Read the model definition and answer for the solid it produces. Units are mm, in the model's axes. Face numbers are marked on the shaded views. A direction names the side the tool comes from. Coordinates: 2 decimals unless noted, no trailing zeros. Write each loop counter-clockwise with the first axis right and the second up, starting at its lowest first coordinate (ties: lowest second). Pieces come first, ordered by that corner, then holes.
(1) The part is cut by section B-B, the plane y = 38. State how many separate pieces and enclosed holes the cut face has, and give its area (3 significant figures).
(2) The part is cut by section A-A, the plane z = 255. Determine the outline of the cut face in (x, y), and give its area (3 significant figures).
(3) Straight lines are drawn through the part: line 1 along Z through (x, y) = (65, 22); line 2 along Z through (x, y) = (63, 25.5); line 3 along X through (y, z) = (31, 65). For each, find the intervals that lie inside material, in ascending order.
(4) Which of the six approach directions +Z, -Z, +X, -X, +Y, -Y give full straight-line access (tool end or side, diameter ignored) to the marked faces 4, 5 and 6?
(5) Given pin 1 (12 mm diameter, centred on x = 13.5, y = 34.5, fed in from -Z); pin 2 (3 mm diameter, centred on x = 95.5, y = 44, fed in from +Z); pin 3 (8 mm diameter, centred on y = 66.5, z = 295.5, fed in from +X), each flat-ended and moving along its own axis, determine where each tip first touches the part or whether it passes through.
(6) Determine the mould class of the marked faces 1, 2 and 3 for opening direction Z: pulls with the +Z half, pulls with the -Z half, needs draft (parallel to the pull), parting line crosses it, or undercut.
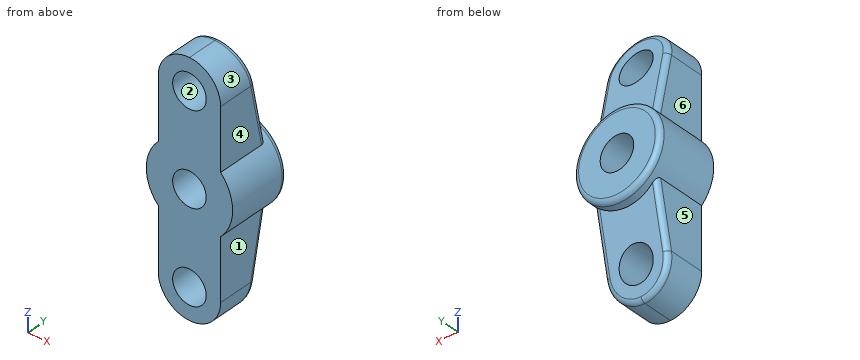
Autodesk Inventor part; units mm, degrees
ref_plane "YZ Plane" through (0, 0, 0) normal (1, 0, 0) x (0, 1, 0)
ref_plane "XZ Plane" through (0, 0, 0) normal (0, 1, 0) x (-1, 0, 0)
ref_plane "XY Plane" through (0, 0, 0) normal (0, 0, 1) x (1, 0, 0)
sketch "Sketch5" plane through (0, 0, 0) normal (1, 0, 0) x (0, 1, 0)
  line L0 (0, 0) -> (0, 510)
  line L1 (0, 510) -> (70, 510)
  line L2 (70, 510) -> (70, 0)
  line L3 (70, 0) -> (0, 0)
  line L4 (0, 255) -> (110, 255)
  line L5 (110, 255) -> (110, 315)
  line L6 (110, 315) -> (70, 510)
  line L7 (110, 255) -> (110, 195)
  line L8 (110, 195) -> (70, 0)
  line L9 (0, 345) -> (0, 255)
  dimension "d9" = 510
  dimension "d10" = 70
  dimension "d11" = 510
  dimension "d12" = 110
  dimension "d13" = 60
  dimension "d14" = 60
extrude "Extrusion4" add sketch "Sketch5" along normal blind 130
fillet "Fillet1" radius 65 4 edges at (130, 35, 510) (0, 35, 510) (130, 35, 0) (0, 35, 0)
sketch "Sketch7" plane through (0, 0, 65) normal (0, -1, 0) x (1, 0, 0)
  line L0 (0, -65) -> (0, 190)
  line L1 (0, 130) -> (0, 250)
  line L2 (0, 190) -> (65, 190)
  circle A0 centre (65, 190) radius 90
  dimension "d28" = 65
  dimension "d29" = 180
extrude "Extrusion6" add sketch "Sketch7" against normal blind 130
sketch "Sketch8" plane through (65, 130, 255) normal (0, 1, 0) x (1, 0, 0)
  circle A0 centre (0, 0) radius 35
  arc A1 (65, 190) -> (-65, 190) centre (0, 190) ccw
  circle A2 centre (0, 190) radius 35
  arc A3 (-65, -190) -> (65, -190) centre (0, -190) ccw
  circle A4 centre (0, -190) radius 35
  point P0 (-65, 255)
  dimension "d32" = 70
  dimension "d39" = 70
  dimension "d40" = 70
extrude "Extrusion7" cut sketch "Sketch8" against normal blind 130
thread "Thread1"
fillet "Fillet2" radius 10 1 edges at (-25, 130, 255)
fillet "Fillet3" radius 10 6 edges at (110.962, 73.9052, 490.962) (0, 96.4359, 381.1248) (130, 96.4359, 381.1248) (110.962, 73.9052, 19.038) (0, 96.4359, 128.8752) (130, 96.4359, 128.8752)
properties part number "Base Superior"
Computed:
1. separate pieces: 1
1. enclosed holes: 3
1. area: 55,400 mm2
2. outline: (-25, 0) - (30, 0) - (30, 130) - (-15, 130) arc R10 ccw to (-25, 120) - close; (100, 0) - (155, 0) - (155, 120) arc R10 ccw to (145, 130) - (100, 130) - close
2. area: 14,300 mm2
3. line 1: z = 0 to 30, 100 to 220, 290 to 410, 480 to 510
3. line 2: z = 0.03 to 30.06, 99.94 to 220.06, 289.94 to 410.06, 479.94 to 509.97
3. line 3: x = 0 to 30, 100 to 130
4. face 4: +Z, +X, +Y, -Y
4. face 5: -Z, -X, +Y, -Y
4. face 6: +Z, -X, +Y, -Y
5. pin 1: stops at z = 18.58
5. pin 2: stops at z = 503.17
5. pin 3: stops at x = 147.27
6. face 1: needs draft
6. face 2: undercut
6. face 3: pulls with the +Z half
